```python
from build123d import *

# Parameters (mm, degrees)
BOSS_EXTRUDE1_DEPTH = 5
CUT_EXTRUDE1_DEPTH  = 150
SKETCH3_R           = 1.5
CUT_EXTRUDE2_DEPTH  = 140.401680724


with BuildPart() as part:
    # Sketch1 → Boss-Extrude1 (new body)
    with BuildSketch(Plane(origin=(0, 0, 0), x_dir=(1, 0, 0), z_dir=(0, 1, 0))):
        with BuildLine():
            Line((64.270386266, 57.510729614), (94.270386266, 57.510729614))
            ThreePointArc((94.270386266, 57.510729614), (101.341454078, 54.581797426), (104.270386266, 47.510729614))
            Line((104.270386266, 47.510729614), (104.270386266, -82.489270386))
            ThreePointArc((104.270386266, -82.489270386), (101.341454078, -89.560338198), (94.270386266, -92.489270386))
            Line((94.270386266, -92.489270386), (64.270386266, -92.489270386))
            Line((64.270386266, -92.489270386), (64.270386266, -67.489270386))
            Line((64.270386266, -67.489270386), (14.270386266, -67.489270386))
            Line((14.270386266, -67.489270386), (14.270386266, -92.489270386))
            Line((14.270386266, -92.489270386), (-55.729613734, -92.489270386))
            Line((-55.729613734, -92.489270386), (-55.729613734, -67.489270386))
            Line((-55.729613734, -67.489270386), (-105.729613734, -67.489270386))
            Line((-105.729613734, -67.489270386), (-105.729613734, -92.489270386))
            Line((-105.729613734, -92.489270386), (-135.729613734, -92.489270386))
            ThreePointArc((-135.729613734, -92.489270386), (-142.800681546, -89.560338198), (-145.729613734, -82.489270386))
            Line((-145.729613734, -82.489270386), (-145.729613734, 47.510729614))
            ThreePointArc((-145.729613734, 47.510729614), (-142.800681546, 54.581797426), (-135.729613734, 57.510729614))
            Line((-135.729613734, 57.510729614), (-105.729613734, 57.510729614))
            Line((-105.729613734, 57.510729614), (-105.729613734, 32.510729614))
            Line((-105.729613734, 32.510729614), (-55.729613734, 32.510729614))
            Line((-55.729613734, 32.510729614), (-55.729613734, 57.510729614))
            Line((-55.729613734, 57.510729614), (14.270386266, 57.510729614))
            Line((14.270386266, 57.510729614), (14.270386266, 32.510729614))
            Line((14.270386266, 32.510729614), (64.270386266, 32.510729614))
            Line((64.270386266, 32.510729614), (64.270386266, 57.510729614))
        make_face()
    extrude(amount=BOSS_EXTRUDE1_DEPTH)

    # Sketch2 → Cut-Extrude1 (cut)
    with BuildSketch(Plane(origin=(0, 0, -57.510729614), x_dir=(-1, 0, 0), z_dir=(0, 0, -1))):
        Polygon((20.729613734, 2.5), (20.729613734, 5), (55.729613734, 5), (105.729613734, 5), (135.729613734, 5), (145.729613734, 5), (145.729613734, 0), (135.729613734, 0), (105.729613734, 0), (55.729613734, 0), (27.729613734, 0), (27.729613734, 2.5), align=None)
    extrude(amount=-CUT_EXTRUDE1_DEPTH, mode=Mode.SUBTRACT)

    # Sketch3 → Cut-Extrude2 (cut, through all)
    with BuildSketch(Plane(origin=(0, 2.5, 0), x_dir=(1, 0, 0), z_dir=(0, 1, 0))):
        with Locations(Location((-24.229613734, -17.489270386, 0), (0, 0, 270))):
            Circle(SKETCH3_R)
        with Locations(Location((-24.229613734, 52.510729614, 0), (0, 0, 270))):
            Circle(SKETCH3_R)
        with Locations(Location((-24.229613734, -87.489270386, 0), (0, 0, 270))):
            Circle(SKETCH3_R)
    extrude(amount=-CUT_EXTRUDE2_DEPTH, mode=Mode.SUBTRACT)


solid = part.part
```
Geometry: final body of the model. Coordinates: model frame, mm. A direction names the side the tool comes from. Coordinates: 2 decimals unless noted, no trailing zeros. Order: outer loops, then holes, each group sorted by start corner. A loop starts at its lowest first (then second) coordinate and runs counter-clockwise, first axis right, second up. Notation, with made-up numbers: (20.25, -34) - (30.25, -34) arc R19 cw to (30.25, -24) - close; hole circle Ø9 at (-14.75, -24.5). An arc over 180 degrees is marked (long way). Write each question's results on one line, items separated by ' | '.
1) Section C-C, the plane z = 32. Return loops of the section in (x, y).
Results list:
outline: (-27.73, 0) - (104.27, 0) - (104.27, 5) - (-20.73, 5) - (-20.73, 2.5) - (-27.73, 2.5) - close
2) Section B-B, the plane y = 3.9. Return loops of the section in (x, z).
Results list:
outline: (-20.73, -57.51) - (14.27, -57.51) - (14.27, -32.51) - (64.27, -32.51) - (64.27, -57.51) - (94.27, -57.51) arc R10 ccw to (104.27, -47.51) - (104.27, 82.49) arc R10 ccw to (94.27, 92.49) - (64.27, 92.49) - (64.27, 67.49) - (14.27, 67.49) - (14.27, 92.49) - (-20.73, 92.49) - close
3) Set-up query: faces 5 (the flat face through (79, 2, -57.511)), 6 (the flat face through (-26, 2.5, 16)), 7 (the flat face through (40, 2, 67.489)), 8 (the flat face through (39, 2, -32.511)), 9 (the cylindrical face through (101.4, 2.5, 89.5)). Return all of +Z, -Z, +X, -X, +Y, -Y with unobstructed straight access to the full face (end or side cutting, diameter ignored); none if empty.
Results list:
face 5: -Z, +X, -X, +Y, -Y | face 6: +Z, -Z, -X, +Y | face 7: +Z, +Y, -Y | face 8: -Z, +Y, -Y | face 9: +Z, +X, +Y, -Y
4) Pull-direction query (X, two-part tool) for faces 1 (the flat face through (14.27, 2, 80)), 2 (the flat face through (104.27, 2, 17)), 3 (the flat face through (64.27, 2, -45)), 4 (the flat face through (43, 5, 16)); classes: pulls with the +X half, pulls with the -X half, needs draft (parallel to the pull), parting line crosses it, or undercut.
Results list:
face 1: undercut | face 2: pulls with the +X half | face 3: undercut | face 4: needs draft
5) Section D-D, the plane x = 20.5. Return loops of the section in (y, z).
Results list:
outline: (0, -32.51) - (5, -32.51) - (5, 67.49) - (0, 67.49) - close
6) Section A-A, the plane z = -43. Return loops of the section in (x, y).
Results list:
outline: (-27.73, 0) - (14.27, 0) - (14.27, 5) - (-20.73, 5) - (-20.73, 2.5) - (-27.73, 2.5) - close; (64.27, 0) - (104.27, 0) - (104.27, 5) - (64.27, 5) - close
7) Line query: line 1 (X direction, y = 1.15, z = 71.5); line 2 (Z direction, x = 63.5, y = 1.25); line 3 (Z direction, x = 94.5, y = 4.1). Output: solid intervals per line, ascending. Write a range as from..to.
Results list:
line 1: -27.73..14.27, 64.27..104.27 | line 2: -32.51..67.49 | line 3: -57.51..92.49
